Geometry: final body of the model. Coordinates: model frame, mm. Face numbers are marked on the shaded views. A direction names the side the tool comes from. Coordinates: 2 decimals unless noted, no trailing zeros. Order: outer loops, then holes, each group sorted by start corner. A loop starts at its lowest first (then second) coordinate and runs counter-clockwise, first axis right, second up. Notation, with made-up numbers: (57.5, 25.25) - (96.5, 25.25) arc R25 cw to (96.5, 47.25) - close; hole circle Ø6 at (12.25, 44.25). An arc over 180 degrees is marked (long way). Use a Markdown table: item, result. Add a question column.
```python
from build123d import *

# Parameters (mm, degrees)
F0_R     = 27.577165
F1_DEPTH = 10
F2_R     = 5
F3_DEPTH = 95
F4_W     = 96.332805
F4_H     = 41.888617
F5_DEPTH = 25


with BuildPart() as f1:
    # F0 (on Front) → F1 (new body)
    with BuildSketch(Plane.XZ):
        with Locations((-28.350001, 23.400001)):
            Circle(F0_R)
    extrude(amount=F1_DEPTH)

    # F2 (on Front) → F3 (join)
    with BuildSketch(Plane.XZ):
        with Locations((-27.377238, 20.944308)):
            Circle(F2_R)
    extrude(amount=F3_DEPTH)

    # F4 (on face) → F5 (join)
    with BuildSketch(Plane.XZ.offset(95)):
        with Locations((-27.377238, 20.944308)):
            Rectangle(F4_W, F4_H)
    extrude(amount=F5_DEPTH)


solid = f1.part
```
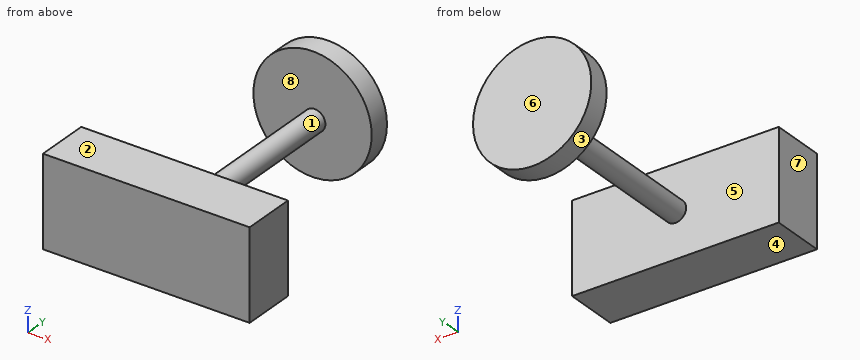
1) Section B-B (x = -28.35). Return loops of the section in (y, z).
2) Pin query (flat end, axial travel): pin 1 (7.5 mm diameter, centred on x = -41, y = -103, fed in from +Z); pin 2 (10 mm diameter, centred on y = -24.5, z = 18.5, fed in from -X); pin 3 (1.5 mm diameter, centred on x = -30.5, z = 5, fed in from +Y); pin 4 (20 mm diameter, centred on x = -32, y = -110.5, fed in from -Z). Return the tip coordinate at first contact, or that it passes through.
3) Section D-D (y = -97). Return loops of the section in (x, z).
4) Section C-C (x = -16.5). Return loops of the section in (y, z).
5) Section A-A (z = 8). Return loops of the section in (x, y), then the cut area to 3 significant figures.
6) Set-up query: the marked faces 1, 2, 3 and 4. Return all of +Z, -Z, +X, -X, +Y, -Y with unobstructed straight access to the full face (end or side cutting, diameter ignored); none if empty.
7) Draft query along Y for the marked faces 5, 6, 7 and 8. Return one class per face: pulls with the +Y half, pulls with the -Y half, needs draft (parallel to the pull), parting line crosses it, or undercut.
8) Ray query, line 1 along Y through (x, z) = (-45, 35.5); line 2 along Y through (x, z) = (-40.5, 46); line 3 along Y through (x, z) = (-62.5, 28.5). Return the intervals inside material, ascending.
Values follow:
| question | item | result |
|---|---|---|
| 1 | outline | (-120, 0) - (-95, 0) - (-95, 16.04) - (-10, 16.04) - (-10, -4.18) - (0, -4.18) - (0, 50.98) - (-10, 50.98) - (-10, 25.85) - (-95, 25.85) - (-95, 41.89) - (-120, 41.89) - close |
| 2 | pin 1 | stops at z = 41.89 |
| 2 | pin 2 | stops at x = -32.38 |
| 2 | pin 3 | stops at y = 0 |
| 2 | pin 4 | stops at z = 0 |
| 3 | outline | (-75.54, 0) - (20.79, 0) - (20.79, 41.89) - (-75.54, 41.89) - close |
| 4 | outline | (-120, 0) - (-95, 0) - (-95, 41.89) - (-120, 41.89) - close; (-10, -1.5) - (0, -1.5) - (0, 48.3) - (-10, 48.3) - close |
| 5 | outline | (-75.54, -120) - (20.79, -120) - (20.79, -95) - (-75.54, -95) - close; (-51.23, -10) - (-5.47, -10) - (-5.47, 0) - (-51.23, 0) - close |
| 5 | area | 2,870 mm² |
| 6 | face 1 | none |
| 6 | face 2 | +Z, +X, -X, -Y |
| 6 | face 3 | +Y |
| 6 | face 4 | -Z, +X, -X, -Y |
| 7 | face 5 | undercut |
| 7 | face 6 | pulls with the +Y half |
| 7 | face 7 | needs draft |
| 7 | face 8 | undercut |
| 8 | line 1 | y = -120 to -95, -10 to 0 |
| 8 | line 2 | y = -10 to 0 |
| 8 | line 3 | y = -120 to -95 |
